Can you work these out from the model? Positions are in its coordinate system, mm. A direction names the side the tool comes from. Round coordinates to 2 decimals unless told otherwise and drop trailing zeros. Loops run counter-clockwise (first coordinate to the right, second up) from the corner with the lowest first, then second, coordinate; pieces in that order, holes last. Notation, with made-up numbers: M 70.25,29 L 79.25,29 A20 cw 79.25,36 Z; hole C 15.25,32 d10. An arc over 180 degrees is marked long. Answer as CSV lines item,"result".
from build123d import *

# Parameters (mm, degrees)
SKETCH1_R           = 2.55
BOSS_EXTRUDE1_DEPTH = 4


with BuildPart() as part:
    # Sketch1 → Boss-Extrude1 (new body)
    with BuildSketch(Plane.XY):
        with BuildLine():
            Line((14.872885109, 17.599965411), (12.706250758, 42.361500851))
            Line((12.706250758, 42.361500851), (12.474619372, 45.008716695))
            Line((12.474619372, 45.008716695), (12.474619372, 47))
            Line((12.474619372, 47), (32.474619372, 47))
            Line((32.474619372, 47), (32.474619372, 45))
            Line((32.474619372, 45), (162.509181482, 14.606317485))
            ThreePointArc((162.509181482, 14.606317485), (174.095167783, 0), (162.509181482, -14.606317485))
            Line((162.509181482, -14.606317485), (32.810836001, -44.921414266))
            ThreePointArc((32.810836001, -44.921414266), (32.472346424, -44.980326678), (32.129340765, -45.000150484))
            Line((32.129340765, -45.000150484), (12.474619372, -45.008716695))
            Line((12.474619372, -45.008716695), (12.706250758, -42.361500851))
            Line((12.706250758, -42.361500851), (14.872885109, -17.599965411))
            ThreePointArc((14.872885109, -17.599965411), (15.740145918, -15.740145918), (17.599965411, -14.872885109))
            Line((17.599965411, -14.872885109), (42.361500851, -12.706250758))
            ThreePointArc((42.361500851, -12.706250758), (44.311843411, -11.744427787), (45.1, -9.717669606))
            Line((45.1, -9.717669606), (45.1, 9.717669606))
            ThreePointArc((45.1, 9.717669606), (44.311843411, 11.744427787), (42.361500851, 12.706250758))
            Line((42.361500851, 12.706250758), (17.599965411, 14.872885109))
            ThreePointArc((17.599965411, 14.872885109), (15.740145918, 15.740145918), (14.872885109, 17.599965411))
        make_face()
        with Locations((159.095167783, 0)):
            Circle(SKETCH1_R, mode=Mode.SUBTRACT)
        with Locations((90, 0)):
            Circle(SKETCH1_R, mode=Mode.SUBTRACT)
    extrude(amount=BOSS_EXTRUDE1_DEPTH)


solid = part.part
Item 1: On a 3-axis mill with a long thin cutter (end or side, diameter ignored), from which of +Z, -Z, +X, -X, +Y, -Y can I reach the whole of each face in a straight line? I mean faces 1 (the face through (29.807, -13.805, 1.972)), 2 (the face through (174.093, 0.282, 1.972)). Say none if no direction works.
Output:
face 1,"+Z, -Z, -X"
face 2,"+Z, -Z, +X"
Item 2: If we section it at D-D on x = 59: Write out the boundary of the cut face in (y, z), then the cut area to 3 significant figures.
Output:
outline,"M -38.8,0 L 38.8,0 L 38.8,4 L -38.8,4 Z"
area,"310 mm2"
Item 3: If I drill on line 1 along Y through (x, z) = (21, 3.05) (3 decimals); line 2 along Y through (x, z) = (22.5, 2.9); line 3 along Y through (x, z) = (99.5, 1.4), over which ranges is the centre line in solid material (lowest first)? Write a range as from..to.
Output:
line 1,"y = -45.005..-14.575, 14.575..47"
line 2,"y = -45..-14.44, 14.44..47"
line 3,"y = -29.33..29.33"
Item 4: We'd pull the mould along Y, two halves only. Please class faces 3 (the face through (98.57, -29.55, 1.97)), 4 (the face through (76, 2, 0)), 5 (the face through (44.333, 11.721, 1.972)): released by +Y, released by -Y, zero draft, split by the parting line, or undercut.
Output:
face 3,"released by -Y"
face 4,"zero draft"
face 5,"undercut"
Item 5: If we section it at A-A on y = 0: Write out the boundary of the cut face in (x, z), then the cut area to 3 significant figures.
Output:
outline,"M 45.1,0 L 87.45,0 L 87.45,4 L 45.1,4 Z; M 92.55,0 L 156.55,0 L 156.55,4 L 92.55,4 Z; M 161.65,0 L 174.1,0 L 174.1,4 L 161.65,4 Z"
area,"475 mm2"
Item 6: Will these pins go through, and if not, where does the flat tip stop? pin 1 (2 mm diameter, centred on y = -2, z = 2, fed in from -X); pin 2 (1 mm diameter, centred on y = 46, z = 1, fed in from +X); pin 3 (2 mm diameter, centred on y = 5.5, z = 2, fed in from +X).
Output:
pin 1,"stops at x = 45.1"
pin 2,"stops at x = 32.47"
pin 3,"stops at x = 173.4"
Item 7: If we section it at C-C on x = 90: Write out the boundary of the cut face in (y, z), then the cut area to 3 significant figures.
Output:
outline,"M -31.55,0 L -2.55,0 L -2.55,4 L -31.55,4 Z; M 2.55,0 L 31.55,0 L 31.55,4 L 2.55,4 Z"
area,"232 mm2"
Item 8: If we section it at B-B on z = 0.85: Write out the boundary of the cut face in (x, y), then the cut area to 3 significant figures.
Output:
outline,"M 12.47,-45.01 L 32.13,-45 A3 ccw 32.81,-44.92 L 162.51,-14.61 A15 ccw 162.51,14.61 L 32.47,45 L 32.47,47 L 12.47,47 L 12.47,45.01 L 14.87,17.6 A3 ccw 17.6,14.87 L 42.36,12.71 A3 cw 45.1,9.72 L 45.1,-9.72 A3 cw 42.36,-12.71 L 17.6,-14.87 A3 ccw 14.87,-17.6 Z; hole C 90,0 d5.1; hole C 159.1,0 d5.1"
area,"8,820 mm2"
